For this review, use the dimensioned drawing (mm, ordinates from the lowest corner) and the shaded views. Round coordinates to 2 decimals unless told otherwise and drop trailing zeros. Loops run counter-clockwise (first coordinate to the right, second up) from the corner with the lowest first, then second, coordinate; pieces in that order, holes last. Notation, with made-up numbers: (2.5, 80) - (42.5, 80) arc R17 cw to (42.5, 101) - close; hole circle Ø6 at (-26.75, 27). An arc over 180 degrees is marked (long way). Answer as CSV lines item,"result". Start each with the question number.
(1) Consider section A-A (y = 2.5). Give the boundary of the cut face in (x, z).
(2) For P1, Ø1, axis at y = 2.5, z = 19.5, coming from the -X side, flat-tipped, find the tip position at first contact; note if it passes through.
(3) Consider section C-C (y = 11.25). Give the boundary of the cut face in (x, z), and give its area (3 significant figures).
(4) Consider section B-B (z = 4). Give the boundary of the cut face in (x, y), and give its area (3 significant figures).
(5) Wall thickness on L1, parallel to X at y = 14, z = 12: over which ranges is the line inside the solid? List them lowest first.
(6) Consider section D-D (z = 12.5). Give the boundary of the cut face in (x, y).
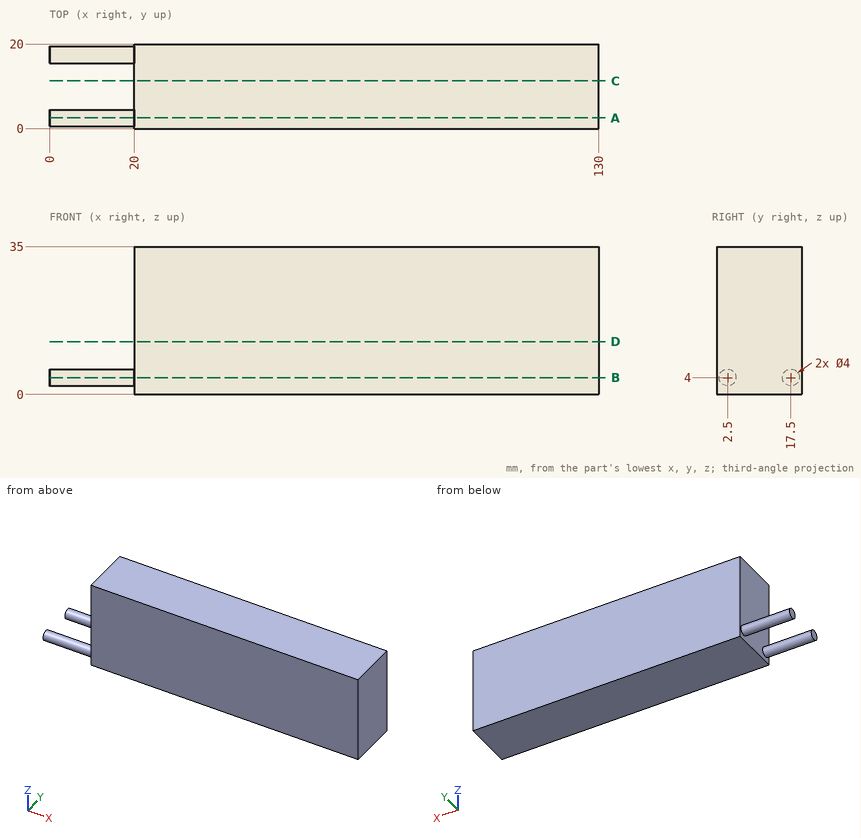
Determined:
1,outline,"(0, 2) - (20, 2) - (20, 0) - (130, 0) - (130, 35) - (20, 35) - (20, 6) - (0, 6) - close"
2,P1,"stops at x = 20"
3,outline,"(20, 0) - (130, 0) - (130, 35) - (20, 35) - close"
3,area,"3,850 mm^2"
4,outline,"(0, 0.5) - (20, 0.5) - (20, 0) - (130, 0) - (130, 20) - (20, 20) - (20, 19.5) - (0, 19.5) - (0, 15.5) - (20, 15.5) - (20, 4.5) - (0, 4.5) - close"
4,area,"2,360 mm^2"
5,L1,"x = 20 to 130"
6,outline,"(20, 0) - (130, 0) - (130, 20) - (20, 20) - close"
